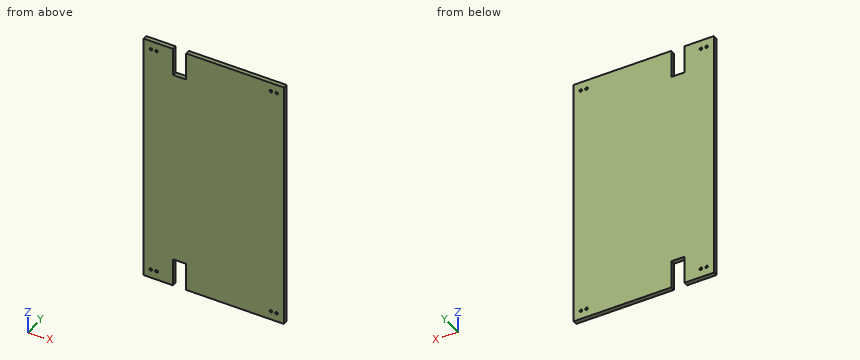
Autodesk Inventor part; units mm, degrees
ref_plane "YZ Plane" through (0, 0, 0) normal (1, 0, 0) x (0, 1, 0)
ref_plane "XZ Plane" through (0, 0, 0) normal (0, 1, 0) x (-1, 0, 0)
ref_plane "XY Plane" through (0, 0, 0) normal (0, 0, 1) x (1, 0, 0)
sketch "Esquisse1" plane through (0, 0, 0) normal (0, 1, 0) x (-1, 0, 0)
  line L0 (94.7405, 132.2434) -> (-66.7595, 132.2434)
  line L1 (-66.7595, 132.2434) -> (-66.7595, -157.7566)
  line L2 (-66.7595, -157.7566) -> (94.7405, -157.7566)
  line L3 (94.7405, -157.7566) -> (94.7405, 132.2434)
  point P0 (0, 0)
  dimension "d0" = 290
  dimension "d1" = 161.5
extrude "Extrusion1" add sketch "Esquisse1" along normal blind 5
sketch "Esquisse3" plane through (0, 5, 0) normal (0, 1, 0) x (1, 0, 0)
  circle A0 centre (58.2595, 147.7566) radius 1.5
  circle A1 centre (51.7595, 147.7566) radius 1.5
  circle A2 centre (58.2595, -122.2434) radius 1.5
  circle A3 centre (51.7595, -122.2434) radius 1.5
  line L0 (-13.9905, 179.8328) -> (-13.9905, -180.1419)
  line L1 (66.7595, -132.2434) -> (66.7595, 157.7566)
  circle A4 centre (-86.2405, 147.7566) radius 1.5
  circle A5 centre (-79.7405, 147.7566) radius 1.5
  circle A6 centre (-86.2405, -122.2434) radius 1.5
  circle A7 centre (-79.7405, -122.2434) radius 1.5
  point P0 (0, 0)
  dimension "d11" = 80.75
extrude "Extrusion3" cut sketch "Esquisse3" against normal up to next
sketch "Esquisse4" plane through (0, 5, 0) normal (0, 1, 0) x (1, 0, 0)
  line L0 (-94.7405, -132.2434) -> (66.7595, -132.2434)
  line L1 (-60.7405, -100.2434) -> (-45.7405, -100.2434)
  line L2 (-45.7405, -100.2434) -> (-45.7405, -132.2434)
  line L3 (-45.7405, -132.2434) -> (-60.7405, -132.2434)
  line L4 (-60.7405, -132.2434) -> (-60.7405, -100.2434)
  line L5 (-94.7405, 157.7566) -> (-94.7405, -132.2434)
  line L6 (-60.7405, 125.7566) -> (-45.7405, 125.7566)
  line L7 (-45.7405, 125.7566) -> (-45.7405, 157.7566)
  line L8 (-45.7405, 157.7566) -> (-60.7405, 157.7566)
  line L9 (-60.7405, 157.7566) -> (-60.7405, 125.7566)
  line L10 (66.7595, 157.7566) -> (-94.7405, 157.7566)
  point P0 (0, 0)
  dimension "d12" = 15
  dimension "d13" = 32
  dimension "d14" = 34
  dimension "d15" = 34
  dimension "d16" = 15
  dimension "d17" = 32
  dimension "d18" = 0
extrude "Extrusion4" cut sketch "Esquisse4" against normal through all
properties part number "étage"
Can you work these out from the model? Positions are in its coordinate system, mm. Give positions to 0.01 mm unless a question says otherwise; leave off trailing zeros. Write each loop counter-clockwise with the first axis right and the second up, starting at its lowest first coordinate (ties: lowest second). Pieces come first, ordered by that corner, then holes. Notation, with made-up numbers: M -29,3 L -12,3 A21 ccw -12,40 Z; hole C -26,-39 d1. An arc over 180 degrees is marked long. Answer in a Markdown table with one row per item. Add a question column.
Item 1: Imagine slicing it at A-A, the plane x = -48.5. Write out the boundary of the cut face in (y, z).
Item 2: For pin 1 Ø2.5 at (x, y) = (-56, 2.5) entering from +Z; pin 2 Ø2.5 at (x, y) = (-50.5, 1.5) entering from -Z, each with a flat end and sliding along its axis, tell me the tip position at first contact or that it passes through.
Item 3: Please list where these lines run through material, in increasing order: L1, parallel to Z at x = -86.5, y = 4.3; L2, parallel to X at y = 0.6, z = -134.5; L3, parallel to Z at x = 59, y = 3.25.
Item 4: Imagine slicing it at B-B, the plane y = 2.2. State how many separate pieces and enclosed holes the cut face has, plus the area to 3 significant figures.
Evaluation:
| question | item | result |
|---|---|---|
| 1 | outline | M 0,-125.76 L 5,-125.76 L 5,100.24 L 0,100.24 Z |
| 2 | pin 1 | stops at z = 100.24 |
| 2 | pin 2 | stops at z = -125.76 |
| 3 | L1 | z = -157.76 to -149.23, -146.28 to 120.77, 123.72 to 132.24 |
| 3 | L2 | x = -94.74 to -60.74, -45.74 to 66.76 |
| 3 | L3 | z = -157.76 to -149.06, -146.45 to 120.94, 123.55 to 132.24 |
| 4 | separate pieces | 1 |
| 4 | enclosed holes | 8 |
| 4 | area | 45,800 mm² |
